Verification items for the finished model (mm, model axes). A direction names the side the tool comes from. Coordinates: 2 decimals unless noted, no trailing zeros. Order: outer loops, then holes, each group sorted by start corner. A loop starts at its lowest first (then second) coordinate and runs counter-clockwise, first axis right, second up.
Q1. Cross-section at A-A, the plane z = -150. Record the boundary of the cut face in (x, y).
Q2. Set-up check for faces 4 (the flat face through (427.705, -4, -170)), 5 (the flat face through (443.58, -4, 88)), 6 (the flat face through (456, -4, -285.75)): record each of +Z, -Z, +X, -X, +Y, -Y from which the full face is reachable in a straight line by a thin tool's end or side.
Q3. Draft check along X on faces 1 (the flat face through (168, -312.738, 1)), 2 (the flat face through (-140.62, -4, -51)), 3 (the flat face through (-83.47, -4, -173)). Enter one of: pulls with the +X half, pulls with the -X half, needs draft (parallel to the pull), parting line crosses it, or undercut.
Q4. Cross-section at D-D, the plane z = 16.5. Record the boundary of the cut face in (x, y).
Q5. Thickness scan on line 1 (X direction, y = -217.5, z = -195.5); line 2 (Z direction, x = 144, y = -158); line 3 (Z direction, x = 448.5, y = -148). Record the ranges inside material, lowest first.
Q6. Depth check by flat-ended pin: P1, Ø12, axis at y = 178.5, z = 50, coming from the +X side; P2, Ø10, axis at x = 60.5, y = -196, coming from the -Z side. Enter the tip coordinate at first touch or a pass-through.
Q7. Cross-section at B-B, the plane y = 176.5. Record the boundary of the cut face in (x, z), and give its area (3 significant figures).
Q8. Cross-section at C-C, the plane x = 95. Record the boundary of the cut face in (y, z).
from build123d import *

# Parameters (mm, degrees)
F0_W     = 584.2
F0_H     = 177.8
F1_DEPTH = 312.7375


with BuildPart() as f1:
    # F0 (on Front) → F1 (new body, symmetric)
    with BuildSketch(Plane.XZ):
        with Locations((151.479768, 88.9)):
            Rectangle(F0_W, F0_H)
        Polygon((443.579768, 0), (-140.620232, 0), (-140.620232, -285.75), (-83.470232, -285.75), (-83.470232, -57.15), (427.704768, -57.15), (427.704768, -285.75), (484.854768, -285.75), (484.854768, 0), align=None)
    extrude(amount=F1_DEPTH, both=True)


solid = f1.part
Check values:
1. outline: (-140.62, -312.74) - (-83.47, -312.74) - (-83.47, 312.74) - (-140.62, 312.74) - close; (427.7, -312.74) - (484.85, -312.74) - (484.85, 312.74) - (427.7, 312.74) - close
2. face 4: -Z, +Y, -Y
2. face 5: +Z, +X, +Y, -Y
2. face 6: -Z, +X, -X, +Y, -Y
3. face 1: needs draft
3. face 2: pulls with the -X half
3. face 3: undercut
4. outline: (-140.62, -312.74) - (443.58, -312.74) - (443.58, 312.74) - (-140.62, 312.74) - close
5. line 1: x = -140.62 to -83.47, 427.7 to 484.85
5. line 2: z = -57.15 to 177.8
5. line 3: z = -285.75 to 0
6. P1: stops at x = 443.58
6. P2: stops at z = -57.15
7. outline: (-140.62, -285.75) - (-83.47, -285.75) - (-83.47, -57.15) - (427.7, -57.15) - (427.7, -285.75) - (484.85, -285.75) - (484.85, 0) - (443.58, 0) - (443.58, 177.8) - (-140.62, 177.8) - close
7. area: 166,000 mm2
8. outline: (-312.74, -57.15) - (312.74, -57.15) - (312.74, 177.8) - (-312.74, 177.8) - close
